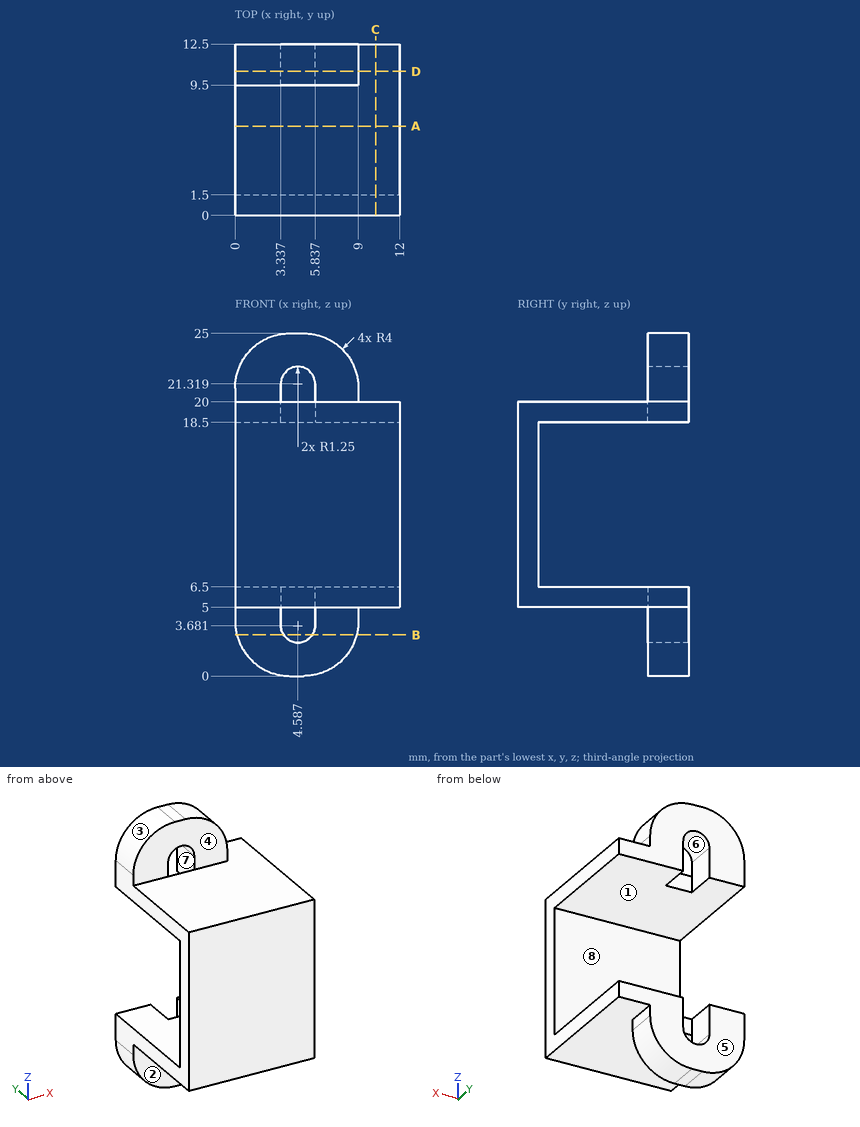
Study the drawing (mm; zero at the part's minimum x, y, z) and answer. A direction names the side the tool comes from. Coordinates: 2 decimals unless noted, no trailing zeros. Write each loop counter-clockwise with the first axis right and the second up, starting at its lowest first coordinate (ties: lowest second). Pieces come first, ordered by that corner, then holes. Notation, with made-up numbers: (32.5, 77) -> (67.5, 77) arc R11 cw to (67.5, 98) -> close; hole circle Ø6 at (-31.5, -23.75). An arc over 180 degrees is marked (long way). Write item = value, one per line.
(1) For a pull along Z with two mould halves and no side action, classify the marked faces 1, 2 and 3 as +Z half, -Z half, draft (parallel to the pull), parting line (faces both ways), or undercut.
From the geometry:
face_1 = undercut
face_2 = draft
face_3 = +Z half
(2) Section C-C on x = 10.25 is taken. Write down the section's boundary in (y, z), plus the area to 3 significant figures.
From the geometry:
outline = (0, 5) -> (12.5, 5) -> (12.5, 6.5) -> (1.5, 6.5) -> (1.5, 18.5) -> (12.5, 18.5) -> (12.5, 20) -> (0, 20) -> close
area = 55.5 mm2
(3) Straight lines are drawn through the part: L1, parallel to Z at x = 10, y = 6.5; L2, parallel to Z at x = 4.5, y = 11; L3, parallel to Y at x = 4.25, z = 17.5. For each, find the intervals that lie inside material, in ascending order. Write a range as from..to.
From the geometry:
L1 = 5..6.5, 18.5..20
L2 = 0..2.43, 22.57..25
L3 = 0..1.5
(4) Section A-A on y = 6.5 is taken. Write down the section's boundary in (x, z).
From the geometry:
outline = (0, 5) -> (12, 5) -> (12, 6.5) -> (0, 6.5) -> close; (0, 18.5) -> (12, 18.5) -> (12, 20) -> (0, 20) -> close
(5) Given pin 1 Ø3 at (x, y) = (7.5, 6.5) entering from +Z; pin 2 Ø0.8 at (y, z) = (11.5, 20.5) entering from +X; pin 3 Ø4 at (y, z) = (8, 15.5) entering from -X; pin 4 Ø1 at (x, z) = (4.5, 11) entering from +Y, each flat-ended and moving along its own axis, determine where each tip first touches the part or whether it passes through.
From the geometry:
pin_1 = 20
pin_2 = 9
pin_3 = through
pin_4 = 1.5
(6) Section B-B on z = 3 is taken. Write down the section's boundary in (x, y) (1 decimal).
From the geometry:
outline = (0.1, 9.5) -> (3.5, 9.5) -> (3.5, 12.5) -> (0.1, 12.5) -> close; (5.6, 9.5) -> (8.9, 9.5) -> (8.9, 12.5) -> (5.6, 12.5) -> close
(7) Which of the six approach directions +Z, -Z, +X, -X, +Y, -Y give full straight-line access (tool end or side, diameter ignored) to the marked faces 4, 5, 6, 7 and 8?
From the geometry:
face_4 = +Z, +X, -X, -Y
face_5 = +Z, -Z, +X, -X, +Y
face_6 = +Y, -Y
face_7 = +Y
face_8 = +X, -X, +Y
(8) Section D-D on y = 10.5 is taken. Write down the section's boundary in (x, z).
From the geometry:
outline = (0, 4) arc R4 ccw to (4, 0) -> (5, 0) arc R4 ccw to (9, 4) -> (9, 5) -> (12, 5) -> (12, 6.5) -> (5.84, 6.5) -> (5.84, 3.68) arc R1.25 cw to (3.34, 3.68) -> (3.34, 6.5) -> (0, 6.5) -> close; (0, 18.5) -> (3.34, 18.5) -> (3.34, 21.32) arc R1.25 cw to (5.84, 21.32) -> (5.84, 18.5) -> (12, 18.5) -> (12, 20) -> (9, 20) -> (9, 21) arc R4 ccw to (5, 25) -> (4, 25) arc R4 ccw to (0, 21) -> close
